Geometry check sheet. Reference: the model listing, model coordinates, mm. Face numbers are marked on the shaded views. A direction names the side the tool comes from. Round coordinates to 2 decimals unless told otherwise and drop trailing zeros. Write each loop counter-clockwise with the first axis right and the second up, starting at its lowest first coordinate (ties: lowest second). Pieces come first, ordered by that corner, then holes. Notation, with made-up numbers: (-32, -23.5) -> (27, -23.5) arc R21 cw to (27, -14.5) -> close; hole circle Ø4 at (-16, 19.5). An arc over 180 degrees is marked (long way). One line per question, with ' | ' between items.
```python
from build123d import *

# Parameters (mm, degrees)
CUT_EXTRUDE_1_DEPTH = 1.04
FILLET_1_R          = 0.1


with BuildPart() as part:
    # 草图1 → 旋转1 (revolve)
    with BuildSketch(Plane.XY):
        with BuildLine():
            Line((0, 2.304545455), (-1.8, 2.304545455))
            ThreePointArc((-1.8, 2.304545455), (-2.467032631, 1.569929856), (-2.85, 0.654545455))
            Line((-2.85, 0.654545455), (-1.5, 0.654545455))
            Line((-1.5, 0.654545455), (-1.5, -24.345454545))
            Line((-1.5, -24.345454545), (0, -24.345454545))
            Line((0, -24.345454545), (0, 2.304545455))
        make_face()
    revolve(axis=Axis((0, 0, 0), (0, 1, 0)))

    # 草图2 → 切除-拉伸1 (cut)
    with BuildSketch(Plane(origin=(0, 2.304545455, 0), x_dir=(1, 0, 0), z_dir=(0, 1, 0))):
        Polygon((0, -1.172021046), (1.015, -0.586010523), (1.015, 0.586010523), (0, 1.172021046), (-1.015, 0.586010523), (-1.015, -0.586010523), align=None)
    extrude(amount=-CUT_EXTRUDE_1_DEPTH, mode=Mode.SUBTRACT)

    # 圆角1
    fillet_1_edges = [part.edges().sort_by_distance(p)[0] for p in [
        (1.5, 0.654545455, 0),
    ]]
    fillet(fillet_1_edges, radius=FILLET_1_R)


solid = part.part
```
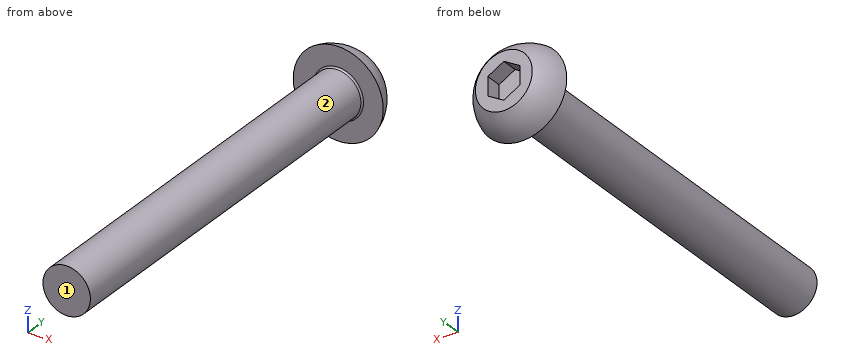
(1) Sectioned sample at C-C on z = -2.2. Record the cut outline in (x, y).
Resolved:
outline: (-1.81, 0.65) -> (1.81, 0.65) arc R1.93 ccw to start
(2) Access from +Z, -Z, +X, -X, +Y, -Y to the whole of each face (thin tool, end or side, straight path). Record for the marked faces 1 and 2.
Resolved:
face 1: +Z, -Z, +X, -X, -Y | face 2: -Y
(3) Sectioned sample at B-B on y = -19.75. Record the cut outline in (x, z).
Resolved:
outline: circle Ø3 at (0, 0)
(4) Go/stop test with flat-tipped pins: pin 1 (1.1 mm diameter, centred on y = 1.5, z = 0, fed in from +X); pin 2 (0.5 mm diameter, centred on y = 2, z = 0, fed in from -X); pin 3 (3 mm diameter, centred on x = 2, y = -7, fed in from -Z). Record where each tip stops, or that it passes through.
Resolved:
pin 1: stops at x = 2.77 | pin 2: stops at x = -2.34 | pin 3: stops at z = -1.41
(5) Sectioned sample at A-A on z = 0. Record the cut outline in (x, y) (3 decimals).
Resolved:
outline: (-2.85, 0.655) -> (-1.6, 0.655) arc R0.1 cw to (-1.5, 0.555) -> (-1.5, -24.345) -> (1.5, -24.345) -> (1.5, 0.555) arc R0.1 cw to (1.6, 0.655) -> (2.85, 0.655) arc R2.924 ccw to (1.8, 2.305) -> (1.015, 2.305) -> (1.015, 1.265) -> (-1.015, 1.265) -> (-1.015, 2.305) -> (-1.8, 2.305) arc R2.924 ccw to start
(6) Material ranges on line 1 (Y direction, x = 0.35, z = -1.65); line 2 (Y direction, x = -0.85, z = -0.1); line 3 (X direction, y = -11.75, z = 1), recorded low to high.
Resolved:
line 1: y = 0.65 to 2.3 | line 2: y = -24.35 to 1.26 | line 3: x = -1.12 to 1.12
